```python
from build123d import *

# Parameters (mm, degrees)
F1_DEPTH = 3
F2_DEPTH = 8
F0_R     = 15
F3_DEPTH = 20
F4_SIZE  = 2


with BuildPart() as f1:
    # F0 (on Top) → F1 (new body)
    with BuildSketch(Plane.XY):
        with BuildLine():
            Line((2, 0), (4, 0))
            ThreePointArc((4, 0), (2.8284271247, 2.8284271247), (0, 4))
            Line((0, 4), (0, 2))
            ThreePointArc((0, 2), (1.4142135624, 1.4142135624), (2, 0))
        make_face()
        with BuildLine():
            Line((0, 2), (0, 4))
            ThreePointArc((0, 4), (-2.8284271247, 2.8284271247), (-4, 0))
            Line((-4, 0), (-2, 0))
            ThreePointArc((-2, 0), (-1.4142135624, 1.4142135624), (0, 2))
        make_face()
        with BuildLine():
            ThreePointArc((-4, 0), (-2.8284271247, -2.8284271247), (0, -4))
            Line((0, -4), (0, -2))
            ThreePointArc((0, -2), (-1.4142135624, -1.4142135624), (-2, 0))
            Line((-2, 0), (-4, 0))
        make_face()
        with BuildLine():
            ThreePointArc((0, -4), (2.8284271247, -2.8284271247), (4, 0))
            Line((4, 0), (2, 0))
            ThreePointArc((2, 0), (1.4142135624, -1.4142135624), (0, -2))
            Line((0, -2), (0, -4))
        make_face()
    extrude(amount=F1_DEPTH)

    # F0 (on Top) → F2 (join)
    with BuildSketch(Plane.XY):
        with BuildLine():
            Line((4, 0), (7.5, 0))
            ThreePointArc((7.5, 0), (5.3033008589, 5.3033008589), (0, 7.5))
            Line((0, 7.5), (0, 4))
            ThreePointArc((0, 4), (2.8284271247, 2.8284271247), (4, 0))
        make_face()
        with BuildLine():
            ThreePointArc((-7.5, 0), (-5.3033008589, -5.3033008589), (0, -7.5))
            Line((0, -7.5), (0, -4))
            ThreePointArc((0, -4), (-2.8284271247, -2.8284271247), (-4, 0))
            Line((-4, 0), (-7.5, 0))
        make_face()
        with BuildLine():
            ThreePointArc((0, -7.5), (5.3033008589, -5.3033008589), (7.5, 0))
            Line((7.5, 0), (4, 0))
            ThreePointArc((4, 0), (2.8284271247, -2.8284271247), (0, -4))
            Line((0, -4), (0, -7.5))
        make_face()
        with BuildLine():
            Line((0, 4), (0, 7.5))
            ThreePointArc((0, 7.5), (-5.3033008589, 5.3033008589), (-7.5, 0))
            Line((-7.5, 0), (-4, 0))
            ThreePointArc((-4, 0), (-2.8284271247, 2.8284271247), (0, 4))
        make_face()
        with BuildLine():
            ThreePointArc((-10, 0), (-7.0710678119, -7.0710678119), (0, -10))
            Line((0, -10), (0, -7.5))
            ThreePointArc((0, -7.5), (-5.3033008589, -5.3033008589), (-7.5, 0))
            Line((-7.5, 0), (-10, 0))
        make_face()
        with BuildLine():
            Line((7.5, 0), (10, 0))
            ThreePointArc((10, 0), (7.0710678119, 7.0710678119), (0, 10))
            Line((0, 10), (0, 7.5))
            ThreePointArc((0, 7.5), (5.3033008589, 5.3033008589), (7.5, 0))
        make_face()
    extrude(amount=F2_DEPTH)

    # F0 (on Top) → F3 (join)
    with BuildSketch(Plane.XY):
        Circle(F0_R)
        with BuildLine():
            ThreePointArc((0, 10), (7.0710678119, 7.0710678119), (10, 0))
            ThreePointArc((10, 0), (7.0710678119, -7.0710678119), (0, -10))
            ThreePointArc((0, -10), (-7.0710678119, -7.0710678119), (-10, 0))
            ThreePointArc((-10, 0), (-7.0710678119, 7.0710678119), (0, 10))
        make_face(mode=Mode.SUBTRACT)
        with BuildLine():
            Line((0, 7.5), (0, 10))
            ThreePointArc((0, 10), (-7.0710678119, 7.0710678119), (-10, 0))
            Line((-10, 0), (-7.5, 0))
            ThreePointArc((-7.5, 0), (-5.3033008589, 5.3033008589), (0, 7.5))
        make_face()
        with BuildLine():
            ThreePointArc((0, -10), (7.0710678119, -7.0710678119), (10, 0))
            Line((10, 0), (7.5, 0))
            ThreePointArc((7.5, 0), (5.3033008589, -5.3033008589), (0, -7.5))
            Line((0, -7.5), (0, -10))
        make_face()
    extrude(amount=F3_DEPTH)

    # F4
    f4_edges = [f1.edges().sort_by_distance(p)[0] for p in [
        (-5.303301, 5.303301, 20),
        (5.303301, -5.303301, 20),
        (7.071068, 7.071068, 20),
        (-7.071068, -7.071068, 20),
    ]]
    chamfer(f4_edges, length=F4_SIZE)


solid = f1.part
```
The model under review builds one solid part; all positions refer to its coordinate system, in mm. A direction names the side the tool comes from. Round coordinates to 2 decimals unless told otherwise and drop trailing zeros. Loops run counter-clockwise (first coordinate to the right, second up) from the corner with the lowest first, then second, coordinate; pieces in that order, holes last.
Item 1: For faces 1 (the face through (3, 0, 0)), 2 (the face through (0, -9, 14)), list the 3-axis set-ups (+Z, -Z, +X, -X, +Y, -Y) from which the entire face can be reached by the end or side of a thin tool; tool diameter is ignored.
Determined:
face 1: -Z, +X, -X, +Y, -Y
face 2: +Z
Item 2: Take a section at B-B (z = 16.75). Write out the cut boundary in (x, y), then the cut area to 3 significant figures.
Determined:
outline: circle Ø30 at (0, 0); hole (-10, 0) arc R10 ccw to (0, -10) - (0, -7.5) arc R7.5 ccw to (7.5, 0) - (10, 0) arc R10 ccw to (0, 10) - (0, 7.5) arc R7.5 ccw to (-7.5, 0) - close
area: 461 mm2
Item 3: Clearance check with flat-ended pins moving along their axes: pin 1 Ø5 at (y, z) = (9, 11.5) entering from +X; pin 2 Ø10 at (x, z) = (11, 17) entering from +Y; pin 3 Ø2.5 at (x, y) = (1, 2) entering from +Z. State where each tip first meets the part, or that it passes through.
Determined:
pin 1: stops at x = 13.52
pin 2: stops at y = 13.75
pin 3: stops at z = 3
Item 4: For line 1 (Z direction, x = -4.25, y = 5.75); line 2 (Y direction, x = -4, z = 9); line 3 (Y direction, x = -2.25, z = 8.5), list the stretches that pass through material, from the lowest coordinate up.
Determined:
line 1: z = 0 to 8
line 2: y = -14.46 to -9.17, 6.34 to 14.46
line 3: y = -14.83 to -9.74, 7.15 to 14.83
Item 5: Take a section at A-A (z = 7.5). Write out the cut boundary in (x, y), then the cut area to 3 significant figures.
Determined:
outline: circle Ø30 at (0, 0); hole circle Ø8 at (0, 0)
area: 657 mm2
Item 6: Mouldability with a two-part tool opening along X and no side actions: class faces 3 (the face through (-7, 7, 20)), 4 (the face through (-14.985, 0.66, 9.86)), 5 (the face through (5.361, -5.245, 12.93)), 6 (the face through (-5.361, 5.245, 12.93)) as released by +X, released by -X, zero draft, split by the parting line, or undercut.
Determined:
face 3: zero draft
face 4: split by the parting line
face 5: undercut
face 6: undercut
